```python
from build123d import *

# Parameters (mm, degrees)
SKETCH_R           = 31
PAD_DEPTH          = 40
SKETCH001_R        = 22.2
POCKET_DEPTH       = 20
SKETCH002_R        = 1.3
PAD001_DEPTH       = 25
POLARPATTERN_COUNT = 16
SKETCH003_W        = 9.8
SKETCH003_H        = 9.8
POCKET001_DEPTH    = 40.001


with BuildPart() as part:
    # Sketch → Pad (new body)
    with BuildSketch(Plane.XY):
        Circle(SKETCH_R)
    extrude(amount=PAD_DEPTH)

    # Sketch001 → Pocket (cut)
    with BuildSketch(Plane.XY.offset(40)):
        Circle(SKETCH001_R)
    extrude(amount=-POCKET_DEPTH, mode=Mode.SUBTRACT)

    # Sketch002 → Pad001 (new body)
    with BuildSketch(Plane.XY.offset(40)):
        with Locations((0, 22.2)):
            Circle(SKETCH002_R)
    pad001 = extrude(amount=-PAD001_DEPTH)

    # PolarPattern: Pad001 ×16 about axis
    polarpattern_axis = Axis((0, 0, 40), (0, 0, 1))
    for i in range(1, POLARPATTERN_COUNT):
        add(pad001.rotate(polarpattern_axis, i * 360 / POLARPATTERN_COUNT))

    # Sketch003 → Pocket001 (cut, through all)
    with BuildSketch(Plane(origin=(0, 0, 0), x_dir=(1, 0, 0), z_dir=(0, 0, -1))):
        Rectangle(SKETCH003_W, SKETCH003_H)
    extrude(amount=-POCKET001_DEPTH, mode=Mode.SUBTRACT)


solid = part.part
```
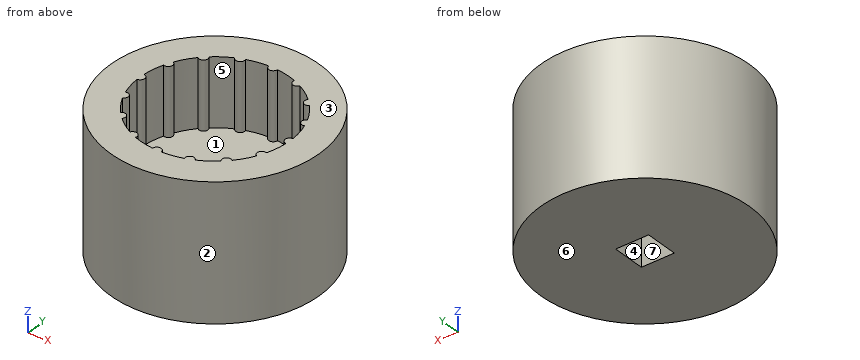
For this review, take the finished solid that the model builds, in its own axes (mm). Face numbers are marked on the shaded views. A direction names the side the tool comes from. Round coordinates to 2 decimals unless told otherwise and drop trailing zeros. Order: outer loops, then holes, each group sorted by start corner. A loop starts at its lowest first (then second) coordinate and runs counter-clockwise, first axis right, second up. Notation, with made-up numbers: (74, 45.5) -> (83, 45.5) arc R16 ccw to (83, 54.5) -> close; hole circle Ø5 at (-12.5, 66). An arc over 180 degrees is marked (long way). Use a Markdown table: item, result.
Item 1: Draft analysis for pull direction X (two halves, no side actions). For the marked faces 1, 2, 3 and 4, state which applies: +X half, -X half, draft (parallel to the pull), parting line (faces both ways), or undercut.
Resolved:
| item | result |
|---|---|
| face 1 | undercut |
| face 2 | parting line |
| face 3 | draft |
| face 4 | undercut |
Item 2: For line 1 along Z through (x, y) = (3.5, -7); line 2 along Y through (x, z) = (13.5, 27); line 3 along Y through (x, z) = (2.5, 16.5), list the stretches that pass through material, from the lowest coordinate up. Write a range as [from, to].
Resolved:
| item | result |
|---|---|
| line 1 | z = [0, 20] |
| line 2 | y = [-27.91, -17.62], [17.62, 27.91] |
| line 3 | y = [-30.9, -4.9], [4.9, 30.9] |
Item 3: Take a section at D-D (z = 15.5). State the section outline as (x, y) points.
Resolved:
| item | result |
|---|---|
| outline | circle Ø62 at (0, 0); hole (-4.9, -4.9) -> (4.9, -4.9) -> (4.9, 4.9) -> (-4.9, 4.9) -> close |
Item 4: Take a section at C-C (y = 4). State the section outline as (x, z) points.
Resolved:
| item | result |
|---|---|
| outline | (-30.74, 0) -> (-4.9, 0) -> (-4.9, 20) -> (-21.84, 20) -> (-21.84, 40) -> (-30.74, 40) -> close; (4.9, 0) -> (30.74, 0) -> (30.74, 40) -> (21.84, 40) -> (21.84, 20) -> (4.9, 20) -> close |
Item 5: Machinability: for the marked faces 5, 6 and 7, which of the approach directions +Z, -Z, +X, -X, +Y, -Y give a long, thin tool a straight path to every point of the face, cutting with its end or side? Answer none if there is none.
Resolved:
| item | result |
|---|---|
| face 5 | +Z |
| face 6 | -Z, +X, -X, +Y, -Y |
| face 7 | +Z, -Z |
Item 6: Take a section at A-A (x = 0). State the section outline as (y, z) points, plus the area to 3 significant figures.
Resolved:
| item | result |
|---|---|
| outline | (-31, 0) -> (-4.9, 0) -> (-4.9, 20) -> (-20.9, 20) -> (-20.9, 40) -> (-31, 40) -> close; (4.9, 0) -> (31, 0) -> (31, 40) -> (20.9, 40) -> (20.9, 20) -> (4.9, 20) -> close |
| area | 1,450 mm² |
Item 7: For pin 1 (11 mm diameter, centred on x = 1.5, z = 10, fed in from +Y); pin 2 (3 mm diameter, centred on y = -2.5, z = 7, fed in from -X); pin 3 (3 mm diameter, centred on y = -9.5, z = 30, fed in from -X); pin 4 (5 mm diameter, centred on y = 1, z = 6.5, fed in from +X), all flat-tipped, find the tip position at first contact; note any pin that passes through.
Resolved:
| item | result |
|---|---|
| pin 1 | stops at y = 31 |
| pin 2 | stops at x = -30.98 |
| pin 3 | stops at x = -29.95 |
| pin 4 | stops at x = 31 |
